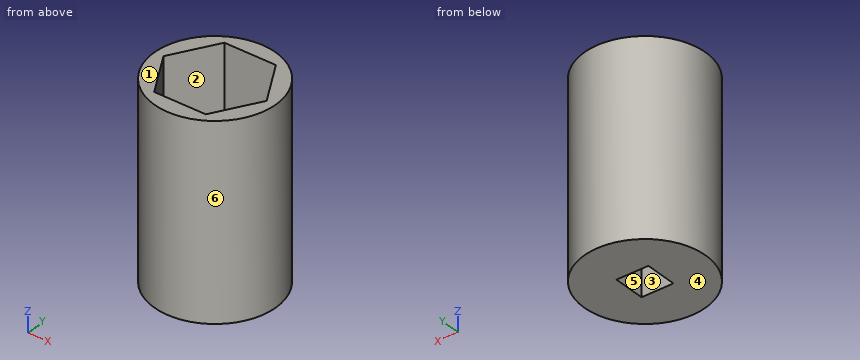
from build123d import *

# Parameters (mm, degrees)
F0_R     = 19
F1_DEPTH = 60
F3_DEPTH = 45
F4_W     = 10
F4_H     = 10
F5_DEPTH = 15


with BuildPart() as f1:
    # F0 (on Top) → F1 (new body)
    with BuildSketch(Plane.XY):
        Circle(F0_R)
    extrude(amount=F1_DEPTH)

    # F2 (on face) → F3 (cut)
    with BuildSketch(Plane.XY.offset(60)):
        Polygon((8.082904, 14), (-8.082904, 14), (-16.165808, 0), (-8.082904, -14), (8.082904, -14), (16.165808, 0), align=None)
    extrude(amount=-F3_DEPTH, mode=Mode.SUBTRACT)

    # F4 (on face) → F5 (cut, through all)
    with BuildSketch(Plane(origin=(0, 0, 0), x_dir=(1, 0, 0), z_dir=(0, 0, -1))):
        Rectangle(F4_W, F4_H)
    extrude(amount=-F5_DEPTH, mode=Mode.SUBTRACT)


solid = f1.part
Verification items for the finished model (mm, model axes). Face numbers are marked on the shaded views. A direction names the side the tool comes from. Coordinates: 2 decimals unless noted, no trailing zeros. Loops run counter-clockwise (first coordinate to the right, second up) from the corner with the lowest first, then second, coordinate; pieces in that order, holes last. Notation, with made-up numbers: (-12.5, 28.25) -> (-4.5, 28.25) arc R25 cw to (-4.5, 48.25) -> close; hole circle Ø6 at (-24.75, -38). An arc over 180 degrees is marked (long way). Answer as a JSON object with one key per item and string values. Group by question number.
Item 1: Sectioned sample at B-B on z = 21.5. Record the boundary of the cut face in (x, y), plus the area to 3 significant figures.
Item 2: Sectioned sample at C-C on y = -2.5. Record the boundary of the cut face in (x, z), plus the area to 3 significant figures.
Item 3: Sectioned sample at A-A on x = 0. Record the boundary of the cut face in (y, z), plus the area to 3 significant figures.
Item 4: Depth check by flat-ended pin: pin 1 (1.5 mm diameter, centred on x = 9, z = 46.5, fed in from -Y); pin 2 (10 mm diameter, centred on x = 14, z = 45, fed in from +Y); pin 3 (5 mm diameter, centred on x = -1, z = 37.5, fed in from +Y). Enter the tip coordinate at first touch or a pass-through.
Item 5: Sectioned sample at D-D on y = 9.5. Record the boundary of the cut face in (x, z), plus the area to 3 significant figures.
Item 6: Scan lines: probe 1 along X at (y, z) = (-6.5, 28); probe 2 along Y at (x, z) = (-3, 23); probe 3 along X at (y, z) = (13.5, 23.5). Record each from-to range of solid material in increasing order.
Item 7: Tool access check on the marked faces 1, 2 and 3. Record the directions out of +Z, -Z, +X, -X, +Y, -Y that give a thin tool (end or side, any length) a straight path to the whole face; none if there is none.
Item 8: Mould release check, pull along X, two halves, no side actions. Record for the marked faces 4, 5 and 6: +X half, -X half, draft (parallel to the pull), parting line (faces both ways), or undercut.
Evaluation:
{
 "1": {"outline": "circle Ø38 at (0, 0); hole (-16.17, 0) -> (-8.08, -14) -> (8.08, -14) -> (16.17, 0) -> (8.08, 14) -> (-8.08, 14) -> close", "area": "455 mm²"},
 "2": {"outline": "(-18.83, 0) -> (-5, 0) -> (-5, 15) -> (-14.72, 15) -> (-14.72, 60) -> (-18.83, 60) -> close; (5, 0) -> (18.83, 0) -> (18.83, 60) -> (14.72, 60) -> (14.72, 15) -> (5, 15) -> close", "area": "785 mm²"},
 "3": {"outline": "(-19, 0) -> (-5, 0) -> (-5, 15) -> (-14, 15) -> (-14, 60) -> (-19, 60) -> close; (5, 0) -> (19, 0) -> (19, 60) -> (14, 60) -> (14, 15) -> (5, 15) -> close", "area": "870 mm²"},
 "4": {"pin 1": "stops at y = -17.12", "pin 2": "stops at y = 16.73", "pin 3": "stops at y = 19"},
 "5": {"outline": "(-16.45, 0) -> (16.45, 0) -> (16.45, 60) -> (10.68, 60) -> (10.68, 15) -> (-10.68, 15) -> (-10.68, 60) -> (-16.45, 60) -> close", "area": "1,010 mm²"},
 "6": {"probe 1": "x = -17.85 to -12.41, 12.41 to 17.85", "probe 2": "y = -18.76 to -14, 14 to 18.76", "probe 3": "x = -13.37 to -8.37, 8.37 to 13.37"},
 "7": {"face 1": "+Z, +X, -X, +Y, -Y", "face 2": "+Z", "face 3": "+Z, -Z"},
 "8": {"face 4": "draft", "face 5": "undercut", "face 6": "parting line"}
}
